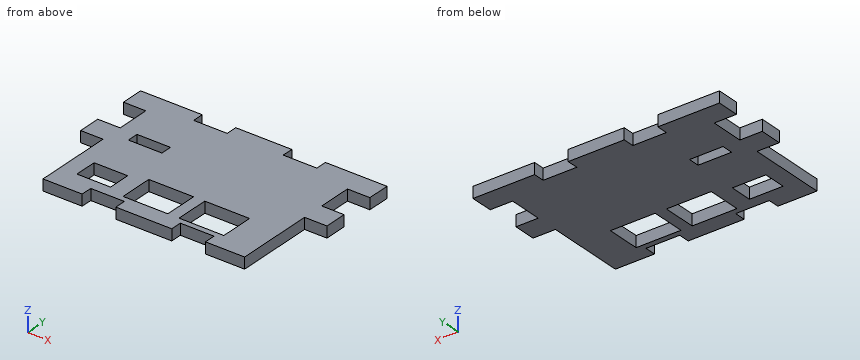
```python
from build123d import *

# Parameters (mm, degrees)
ESQUISSE1_W             = 110
ESQUISSE1_H             = 70
BOSS_EXTRU_1_DEPTH      = 5
ESQUISSE2_W             = 20
ESQUISSE2_H             = 15
ESQUISSE2_W_2           = 15
ESQUISSE2_H_2           = 10
ESQUISSE2_H_3           = 5
ENL_V_MAT_EXTRU_1_DEPTH = 5
ESQUISSE6_W             = 10
ESQUISSE6_H             = 35
ESQUISSE6_H_2           = 15
ESQUISSE6_W_2           = 15
ESQUISSE6_H_3           = 5
ENL_V_MAT_EXTRU_2_DEPTH = 5


with BuildPart() as part:
    # Esquisse1 → Boss.-Extru.1 (new body)
    with BuildSketch(Plane.XY):
        Rectangle(ESQUISSE1_W, ESQUISSE1_H)
    extrude(amount=BOSS_EXTRU_1_DEPTH)

    # Esquisse2 → Enlèv. mat.-Extru.1 (cut)
    with BuildSketch(Plane.XY.offset(5)):
        with Locations((20, -20)):
            Rectangle(ESQUISSE2_W, ESQUISSE2_H)
        with Locations((-5, -20)):
            Rectangle(ESQUISSE2_W, ESQUISSE2_H)
        with Locations((-30, -20)):
            Rectangle(ESQUISSE2_W_2, ESQUISSE2_H_2)
        with Locations((-30, 7.5)):
            Rectangle(ESQUISSE2_W_2, ESQUISSE2_H_3)
    extrude(amount=-ENL_V_MAT_EXTRU_1_DEPTH, mode=Mode.SUBTRACT)

    # Esquisse6 → Enlèv. mat.-Extru.2 (cut)
    with BuildSketch(Plane(origin=(0, 0, 0), x_dir=(-1, 0, 0), z_dir=(0, 0, -1))):
        with Locations((-50, -17.5)):
            Rectangle(ESQUISSE6_W, ESQUISSE6_H)
        with Locations((50, -17.5)):
            Rectangle(ESQUISSE6_W, ESQUISSE6_H)
        with Locations((-50, 17.5)):
            Rectangle(ESQUISSE6_W, ESQUISSE6_H_2)
        with Locations((50, 17.5)):
            Rectangle(ESQUISSE6_W, ESQUISSE6_H_2)
        with Locations((-20, 32.5)):
            Rectangle(ESQUISSE6_W_2, ESQUISSE6_H_3)
        with Locations((20, 32.5)):
            Rectangle(ESQUISSE6_W_2, ESQUISSE6_H_3)
        with Locations((-20, -32.5)):
            Rectangle(ESQUISSE6_W_2, ESQUISSE6_H_3)
        with Locations((20, -32.5)):
            Rectangle(ESQUISSE6_W_2, ESQUISSE6_H_3)
    extrude(amount=-ENL_V_MAT_EXTRU_2_DEPTH, mode=Mode.SUBTRACT)


solid = part.part
```
Can you work these out from the model? Positions are in its coordinate system, mm. Round coordinates to 2 decimals unless told otherwise and drop trailing zeros. Loops run counter-clockwise (first coordinate to the right, second up) from the corner with the lowest first, then second, coordinate; pieces in that order, holes last. Notation, with made-up numbers: M 9.25,1 L 31.25,1 A9 ccw 31.25,8 Z; hole C -7,-14.75 d1. An arc over 180 degrees is marked long. Answer as a JSON object with one key per item and string values. Group by question number.
Q1. Imagine slicing it at C-C, the plane x = -2. Please give me the cut outline in (y, z).
Q2. Please list where these lines run through material, in increasing order: L1, parallel to X at y = -18.5, z = 3.8; L2, parallel to Y at x = -37, z = 3.65; L3, parallel to Y at x = 27, z = 1.55.
Q3. Will these pins go through, and if not, where does the flat tip stop? pin 1 (1 mm diameter, centred on x = -13.5, z = 2.5, fed in from -Y); pin 2 (3 mm diameter, centred on x = -11.5, y = -25.5, fed in from -Z); pin 3 (2.5 mm diameter, centred on y = -18, z = 2, fed in from +X); pin 4 (1.5 mm diameter, centred on x = -48, z = 3.5, fed in from -Y).
Q4. Imagine slicing it at B-B, the plane y = -21. Please give me the cut outline in (x, z), then the cut area to 3 significant figures.
Q5. Imagine slicing it at A-A, the plane x = -32.5. Please give me the cut outline in (y, z).
Q6. Imagine slicing it at D-D, the plane y = 8. Please give me the cut outline in (x, z).
Findings:
{
 "1": {"outline": "M -35,0 L -27.5,0 L -27.5,5 L -35,5 Z; M -12.5,0 L 35,0 L 35,5 L -12.5,5 Z"},
 "2": {"L1": "x = -45 to -37.5, -22.5 to -15, 5 to 10, 30 to 45", "L2": "y = -35 to -25, -15 to 5, 10 to 35", "L3": "y = -30 to -27.5, -12.5 to 30"},
 "3": {"pin 1": "stops at y = -30", "pin 2": "passes through", "pin 3": "stops at x = 45", "pin 4": "stops at y = 0"},
 "4": {"outline": "M -45,0 L -37.5,0 L -37.5,5 L -45,5 Z; M -22.5,0 L -15,0 L -15,5 L -22.5,5 Z; M 5,0 L 10,0 L 10,5 L 5,5 Z; M 30,0 L 45,0 L 45,5 L 30,5 Z", "area": "175 mm2"},
 "5": {"outline": "M -35,0 L -25,0 L -25,5 L -35,5 Z; M -15,0 L 5,0 L 5,5 L -15,5 Z; M 10,0 L 35,0 L 35,5 L 10,5 Z"},
 "6": {"outline": "M -55,0 L -37.5,0 L -37.5,5 L -55,5 Z; M -22.5,0 L 55,0 L 55,5 L -22.5,5 Z"}
}
